from build123d import *

# Parameters (mm, degrees)
SKETCH1_W           = 3.867553816
SKETCH1_H           = 98
BOSS_EXTRUDE3_DEPTH = 20
BOSS_EXTRUDE4_DEPTH = 1.5
CUT_EXTRUDE1_DEPTH  = 54.264192452


with BuildPart() as part:
    # Sketch1 → Boss-Extrude3 (new body)
    with BuildSketch(Plane.XY):
        Rectangle(SKETCH1_W, SKETCH1_H)
    extrude(amount=BOSS_EXTRUDE3_DEPTH)

    # Sketch1<6> → Boss-Extrude4 (add)
    with BuildSketch(Plane.XY):
        with BuildLine():
            Line((1.71, 3.795), (1.71, -3.795))
            ThreePointArc((1.71, -3.795), (0, -5.505), (-1.71, -3.795))
            Line((-1.71, -3.795), (-1.71, 3.795))
            ThreePointArc((-1.71, 3.795), (0, 5.505), (1.71, 3.795))
        make_face()
        with BuildLine():
            Line((1.71, -39.915), (1.71, -47.505))
            ThreePointArc((1.71, -47.505), (0, -49.215), (-1.71, -47.505))
            Line((-1.71, -47.505), (-1.71, -39.915))
            ThreePointArc((-1.71, -39.915), (0, -38.205), (1.71, -39.915))
        make_face()
        with BuildLine():
            Line((1.71, 47.505), (1.71, 39.915))
            ThreePointArc((1.71, 39.915), (0, 38.205), (-1.71, 39.915))
            Line((-1.71, 39.915), (-1.71, 47.505))
            ThreePointArc((-1.71, 47.505), (0, 49.215), (1.71, 47.505))
        make_face()
    extrude(amount=-BOSS_EXTRUDE4_DEPTH)

    # Sketch5 → Cut-Extrude1 (cut, through all)
    with BuildSketch(Plane(origin=(1.933776908, 0, 0), x_dir=(0, 0, -1), z_dir=(1, 0, 0))):
        with BuildLine():
            Line((-13.934698867, 42.838530115), (-13.934698867, -44.584300935))
            ThreePointArc((-13.934698867, -44.584300935), (-14.740439245, -45.390041313), (-15.546179624, -44.584300935))
            Line((-15.546179624, -44.584300935), (-15.546179624, 42.838530115))
            ThreePointArc((-15.546179624, 42.838530115), (-14.740439245, 43.644270494), (-13.934698867, 42.838530115))
        make_face()
        with BuildLine():
            Line((-10.040287038, 42.838530115), (-10.040287038, -44.584300935))
            ThreePointArc((-10.040287038, -44.584300935), (-10.711737354, -45.25575125), (-11.383187669, -44.584300935))
            Line((-11.383187669, -44.584300935), (-11.383187669, 42.838530115))
            ThreePointArc((-11.383187669, 42.838530115), (-10.711737354, 43.509980431), (-10.040287038, 42.838530115))
        make_face()
        with BuildLine():
            Line((-6.548745399, 42.838530115), (-6.548745399, -44.584300935))
            ThreePointArc((-6.548745399, -44.584300935), (-7.220195714, -45.25575125), (-7.891646029, -44.584300935))
            Line((-7.891646029, -44.584300935), (-7.891646029, 42.838530115))
            ThreePointArc((-7.891646029, 42.838530115), (-7.220195714, 43.509980431), (-6.548745399, 42.838530115))
        make_face()
        with BuildLine():
            Line((-2.385753444, 42.838530115), (-2.385753444, -44.584300935))
            ThreePointArc((-2.385753444, -44.584300935), (-3.057203759, -45.25575125), (-3.728654075, -44.584300935))
            Line((-3.728654075, -44.584300935), (-3.728654075, 42.838530115))
            ThreePointArc((-3.728654075, 42.838530115), (-3.057203759, 43.509980431), (-2.385753444, 42.838530115))
        make_face()
    extrude(amount=-CUT_EXTRUDE1_DEPTH, mode=Mode.SUBTRACT)


solid = part.part
Work out the finished part from the listing and answer in its coordinate system (mm). A direction names the side the tool comes from. Give positions to 0.01 mm unless a question says otherwise; leave off trailing zeros. Return JSON: item names as keys, results as strings.
Q1. Each of these flat-tipped pins is pushed along its axis until it touches: pin 1 (1.5 mm diameter, centred on x = -0.5, y = 24, fed in from -Z); pin 2 (1.9 mm diameter, centred on x = 0, z = 6.5, fed in from +Y); pin 3 (1.2 mm diameter, centred on y = 45, z = -1, fed in from +X). Where does it stop, or does it pass through?
Answer below:
{"pin 1": "stops at z = 0", "pin 2": "stops at y = 49", "pin 3": "stops at x = 1.71"}
Q2. Which of the six approach directions +Z, -Z, +X, -X, +Y, -Y give full straight-line access (tool end or side, diameter ignored) to faces 4 (the face through (0, 0, 13.935)), 5 (the face through (1.934, -0.69, 9.86)), 6 (the face through (0, 49, 10)), 7 (the face through (-0.038, -38.205, -0.74)), 8 (the face through (0, 0, -1.5))?
Answer below:
{"face 4": "+X, -X", "face 5": "+Z, -Z, +X, +Y, -Y", "face 6": "+Z, +X, -X, +Y", "face 7": "-Z", "face 8": "-Z, +X, -X, +Y, -Y"}
Q3. Find section A-A, the plane x = 0. State how many separate pieces and enclosed holes the cut face has, and give its area (3 significant figures).
Answer below:
{"separate pieces": "1", "enclosed holes": "4", "area": "1,510 mm^2"}
Q4. Find the intervals of material crossed by line 1 along Z through (x, y) = (1.45, -10); line 2 along Z through (x, y) = (0.05, 3.5); line 3 along Y through (x, z) = (-1.4, 10.75), in increasing order. Write a range as [from, to].
Answer below:
{"line 1": "z = [0, 2.39], [3.73, 6.55], [7.89, 10.04], [11.38, 13.93], [15.55, 20]", "line 2": "z = [-1.5, 2.39], [3.73, 6.55], [7.89, 10.04], [11.38, 13.93], [15.55, 20]", "line 3": "y = [-49, -45.25], [43.51, 49]"}
Q5. The mould has two halves that part along Y. Classify faces 1 (the face through (-1.934, -0.69, 9.86)), 2 (the face through (0.027, 43.644, 14.758)), 3 (the face through (0.038, -49.215, -0.74)): pulls with the +Y half, pulls with the -Y half, needs draft (parallel to the pull), parting line crosses it, or undercut.
Answer below:
{"face 1": "needs draft", "face 2": "undercut", "face 3": "pulls with the -Y half"}
